from build123d import *

# Parameters (mm, degrees)
EXTRUDE_1_DEPTH      = 30
SKETCH_2_R           = 44.45
CUT_EXTRUDE_1_DEPTH  = 4
SKETCH_3_R           = 25.5
SKETCH_3_R_2         = 2.25
CUT_EXTRUDE_2_DEPTH  = 188.619295383
CUT_EXTRUDE_3_DEPTH  = 189.215302247
SKETCH_5_R           = 1.65
CUT_EXTRUDE_4_DEPTH  = 189.215302247
EXTRUDE_START        = -30
EXTRUDE_2_DEPTH      = 30
CUT_EXTRUDE_5_DEPTH  = 198.040604952
CUT_EXTRUDE_7_DEPTH  = 233.432785983
CUT_EXTRUDE_8_DEPTH  = 233.432785983
CUT_EXTRUDE_9_DEPTH  = 233.432785983
FILLET_1_R           = 5
CUT_EXTRUDE_10_DEPTH = 233.432785983
EXTRUDE_START_2      = -5
EXTRUDE_3_DEPTH      = 5
EXTRUDE_4_DEPTH      = 5
SKETCH_14_R          = 4.25
CUT_EXTRUDE_11_DEPTH = 189.364728478
SKETCH_16_W          = 43
SKETCH_16_H          = 30
CUT_EXTRUDE_12_DEPTH = 233.432785983
EXTRUDE_7_REACH      = 188.592
SKETCH_18_W          = 210
SKETCH_18_H          = 5
EXTRUDE_8_DEPTH      = 210
EXTRUDE_9_DEPTH      = 5
EXTRUDE_10_DEPTH     = 5
SKETCH_22_R          = 4.25
CUT_EXTRUDE_13_DEPTH = 187.984035343
FILLET_2_R           = 5
EXTRUDE_11_DEPTH     = 2.5
EXTRUDE_12_DEPTH     = 2.5
CUT_EXTRUDE_15_DEPTH = 5
CUT_EXTRUDE_START    = -5
CUT_EXTRUDE_16_DEPTH = 5


with BuildPart() as part:
    # 草图1 → 凸台-拉伸1 (new body)
    with BuildSketch(Plane(origin=(0, 0, 0), x_dir=(1, 0, 0), z_dir=(0, 1, 0))):
        with BuildLine():
            Line((170, 31.93), (170, -31.93))
            ThreePointArc((170, -31.93), (167.781993847, -38.210172909), (162.111885646, -41.704453387))
            Line((162.111885646, -41.704453387), (15.839142344, -73.308400404))
            ThreePointArc((15.839142344, -73.308400404), (-75, 0), (15.839142344, 73.308400404))
            Line((15.839142344, 73.308400404), (162.111885646, 41.704453387))
            ThreePointArc((162.111885646, 41.704453387), (167.781993847, 38.210172909), (170, 31.93))
        make_face()
    extrude(amount=EXTRUDE_1_DEPTH)

    # 草图2 → 切除-拉伸1 (cut)
    with BuildSketch(Plane(origin=(0, 30, 0), x_dir=(1, 0, 0), z_dir=(0, 1, 0))):
        with Locations(Location((0, 0, 0), (0, 0, 270))):
            Circle(SKETCH_2_R)
    extrude(amount=-CUT_EXTRUDE_1_DEPTH, mode=Mode.SUBTRACT)

    # 草图3 → 切除-拉伸2 (cut, through all)
    with BuildSketch(Plane(origin=(0, 26, 0), x_dir=(1, 0, 0), z_dir=(0, 1, 0))):
        with Locations(Location((0, 0, 0), (0, 0, 270))):
            Circle(SKETCH_3_R)
        with Locations(Location((0, 41, 0), (0, 0, 270))):
            Circle(SKETCH_3_R_2)
        with Locations(Location((28.991378029, 28.991378029, 0), (0, 0, 270))):
            Circle(SKETCH_3_R_2)
        with Locations(Location((41, 0, 0), (0, 0, 270))):
            Circle(SKETCH_3_R_2)
        with Locations(Location((28.991378029, -28.991378029, 0), (0, 0, 270))):
            Circle(SKETCH_3_R_2)
        with Locations(Location((0, -41, 0), (0, 0, 270))):
            Circle(SKETCH_3_R_2)
        with Locations(Location((-28.991378029, -28.991378029, 0), (0, 0, 270))):
            Circle(SKETCH_3_R_2)
        with Locations(Location((-41, 0, 0), (0, 0, 270))):
            Circle(SKETCH_3_R_2)
        with Locations(Location((-28.991378029, 28.991378029, 0), (0, 0, 270))):
            Circle(SKETCH_3_R_2)
    extrude(amount=-CUT_EXTRUDE_2_DEPTH, mode=Mode.SUBTRACT)

    # 草图4 → 切除-拉伸3 (cut, through all)
    with BuildSketch(Plane(origin=(0, 30, 0), x_dir=(1, 0, 0), z_dir=(0, 1, 0))):
        with BuildLine():
            Line((124, 18.5), (134, 18.5))
            ThreePointArc((134, 18.5), (152.5, 0), (134, -18.5))
            Line((134, -18.5), (124, -18.5))
            ThreePointArc((124, -18.5), (105.5, 0), (124, 18.5))
        make_face()
    extrude(amount=-CUT_EXTRUDE_3_DEPTH, mode=Mode.SUBTRACT)

    # 草图5 → 切除-拉伸4 (cut, through all)
    with BuildSketch(Plane(origin=(0, 30, 0), x_dir=(1, 0, 0), z_dir=(0, 1, 0))):
        with Locations(Location((116.75, 25.5, 0), (0, 0, 270))):
            Circle(SKETCH_5_R)
        with Locations(Location((141.25, 25.5, 0), (0, 0, 270))):
            Circle(SKETCH_5_R)
        with Locations(Location((141.25, -25.5, 0), (0, 0, 270))):
            Circle(SKETCH_5_R)
        with Locations(Location((116.75, -25.5, 0), (0, 0, 270))):
            Circle(SKETCH_5_R)
    extrude(amount=-CUT_EXTRUDE_4_DEPTH, mode=Mode.SUBTRACT)

    # 草图6 → 凸台-拉伸2 (add)
    with BuildSketch(Plane(origin=(0, 30, 0), x_dir=(1, 0, 0), z_dir=(0, 1, 0)).offset(EXTRUDE_START)):
        with BuildLine():
            Line((158, 95), (-52, 95))
            Line((-52, 95), (-52, 54.046276467))
            ThreePointArc((-52, 54.046276467), (-20.48558667, 72.148047366), (15.839142344, 73.308400404))
            Line((15.839142344, 73.308400404), (158, 42.592874655))
            Line((158, 42.592874655), (158, 95))
        make_face()
        with BuildLine():
            ThreePointArc((15.839142344, -73.308400404), (-20.48558667, -72.148047366), (-52, -54.046276467))
            Line((-52, -54.046276467), (-52, -95))
            Line((-52, -95), (158, -95))
            Line((158, -95), (158, -42.592874655))
            Line((158, -42.592874655), (15.839142344, -73.308400404))
        make_face()
    extrude(amount=EXTRUDE_2_DEPTH)

    # 草图7 → 切除-拉伸5 (cut, through all)
    with BuildSketch(Plane(origin=(0, 30, 0), x_dir=(1, 0, 0), z_dir=(0, 1, 0))):
        with BuildLine():
            Line((-52, 54.046276467), (-52, -54.046276467))
            ThreePointArc((-52, -54.046276467), (-75, 0), (-52, 54.046276467))
        make_face()
        with BuildLine():
            Line((158, 42.592874655), (158, -42.592874655))
            Line((158, -42.592874655), (162.111885646, -41.704453387))
            ThreePointArc((162.111885646, -41.704453387), (167.781993847, -38.210172909), (170, -31.93))
            Line((170, -31.93), (170, 31.93))
            ThreePointArc((170, 31.93), (167.781993847, 38.210172909), (162.111885646, 41.704453387))
            Line((162.111885646, 41.704453387), (158, 42.592874655))
        make_face()
    extrude(amount=-CUT_EXTRUDE_5_DEPTH, mode=Mode.SUBTRACT)

    # 草图9 → 切除-拉伸7 (cut, through all)
    with BuildSketch(Plane.ZY.offset(52)):
        Polygon((-95, 20), (-60, 10.621778265), (-60, 30), (-95, 30), align=None)
    extrude(amount=-CUT_EXTRUDE_7_DEPTH, mode=Mode.SUBTRACT)

    # 草图10 → 切除-拉伸8 (cut, through all)
    with BuildSketch(Plane.ZY.offset(52)):
        Polygon((-95, 12.753066737), (-52, 1.231251463), (-52, 0), (-95, 0), align=None)
    extrude(amount=-CUT_EXTRUDE_8_DEPTH, mode=Mode.SUBTRACT)

    # 草图8 → 切除-拉伸9 (cut, through all)
    with BuildSketch(Plane.ZY.offset(52)):
        Polygon((0, 0), (52, 0), (52, 17.3), (-52, 17.3), (-52, 0), align=None)
    extrude(amount=-CUT_EXTRUDE_9_DEPTH, mode=Mode.SUBTRACT)

    # 圆角1
    fillet_1_edges = [part.edges().sort_by_distance(p)[0] for p in [
        (53, 10.621778265, -60),
    ]]
    fillet(fillet_1_edges, radius=FILLET_1_R)

    # 草图11 → 切除-拉伸10 (cut, through all)
    with BuildSketch(Plane.ZY.offset(52)):
        Polygon((-95, 12.753066737), (-93.188266684, 19.514547521), (-95, 20), align=None)
    extrude(amount=-CUT_EXTRUDE_10_DEPTH, mode=Mode.SUBTRACT)

    # 草图12 → 凸台-拉伸3 (add)
    with BuildSketch(Plane.ZY.offset(52).offset(EXTRUDE_START_2)):
        with BuildLine():
            Line((-93.188266684, 19.514547521), (-60, 30))
            Line((-60, 30), (-60, 17.137905129))
            ThreePointArc((-60, 17.137905129), (-61.956192855, 13.171138428), (-66.294095226, 12.308275998))
            Line((-66.294095226, 12.308275998), (-93.188266684, 19.514547521))
        make_face()
    extrude(amount=EXTRUDE_3_DEPTH)

    # 草图13 → 凸台-拉伸4 (add)
    with BuildSketch(Plane(origin=(158, 0, 0), x_dir=(0, 0, -1), z_dir=(1, 0, 0))):
        with BuildLine():
            Line((66.294095226, 12.308275998), (93.188266684, 19.514547521))
            Line((93.188266684, 19.514547521), (60, 30))
            Line((60, 30), (60, 17.137905129))
            ThreePointArc((60, 17.137905129), (61.956192855, 13.171138428), (66.294095226, 12.308275998))
        make_face()
    extrude(amount=-EXTRUDE_4_DEPTH)

    # 草图14 → 切除-拉伸11 (cut, through all)
    with BuildSketch(Plane(origin=(0, -5.089745962, -1.36379332), x_dir=(1, 0, 0), z_dir=(0, 0.9659258262890681, 0.2588190451025214))):
        with Locations(Location((-27, 82.063690052, 0), (0, 0, 270))):
            Circle(SKETCH_14_R)
        with Locations(Location((23, 82.063690052, 0), (0, 0, 270))):
            Circle(SKETCH_14_R)
        with Locations(Location((83, 82.063690052, 0), (0, 0, 270))):
            Circle(SKETCH_14_R)
        with Locations(Location((133, 82.063690052, 0), (0, 0, 270))):
            Circle(SKETCH_14_R)
    extrude(amount=-CUT_EXTRUDE_11_DEPTH, mode=Mode.SUBTRACT)

    # 草图16 → 切除-拉伸12 (cut, through all)
    with BuildSketch(Plane.ZY.offset(52)):
        with Locations((73.5, 15)):
            Rectangle(SKETCH_16_W, SKETCH_16_H)
    extrude(amount=-CUT_EXTRUDE_12_DEPTH, mode=Mode.SUBTRACT)

    # 凸台-拉伸7: up to this plane
    extrude_7_end = Plane(origin=(0, -11.851226746, -3.175526636), z_dir=(0, -0.9659258262890681, -0.25881904510252146))
    # 草图18 → 凸台-拉伸7 (add, up to the surface)
    with BuildSketch(Plane(origin=(0, 30, 0), x_dir=(1, 0, 0), z_dir=(0, 1, 0)), mode=Mode.PRIVATE) as extrude_7_sk1:
        with Locations((53, -54.5)):
            Rectangle(SKETCH_18_W, SKETCH_18_H)
    extrude_7_tool1 = split(extrude(extrude_7_sk1.sketch, amount=-EXTRUDE_7_REACH, mode=Mode.PRIVATE), bisect_by=extrude_7_end, keep=Keep.BOTH, mode=Mode.PRIVATE)
    add(extrude_7_tool1.solids().sort_by_distance((53, 30, 54.5))[0])

    # 草图19 → 凸台-拉伸8 (add)
    with BuildSketch(Plane.ZY.offset(52)):
        Polygon((57, -27.975210512), (90.188266684, -36.867979769), (92, -30.106498985), (57, -20.72827725), align=None)
    extrude(amount=-EXTRUDE_8_DEPTH)

    # 草图20 → 凸台-拉伸9 (add)
    with BuildSketch(Plane.ZY.offset(52)):
        Polygon((92, -30.106498985), (57, -20.72827725), (57, 30), align=None)
    extrude(amount=-EXTRUDE_9_DEPTH)

    # 草图21 → 凸台-拉伸10 (add)
    with BuildSketch(Plane(origin=(158, 0, 0), x_dir=(0, 0, -1), z_dir=(1, 0, 0))):
        Polygon((-57, 30), (-92, -30.106498985), (-57, -20.72827725), align=None)
    extrude(amount=-EXTRUDE_10_DEPTH)

    # 草图22 → 切除-拉伸13 (cut, through all)
    with BuildSketch(Plane(origin=(0, -5.089745962, -1.36379332), x_dir=(1, 0, 0), z_dir=(0, 0.9659258262890686, 0.25881904510251946))):
        with Locations(Location((-27, -77.936309948, 0), (0, 0, 270))):
            Circle(SKETCH_22_R)
        with Locations(Location((23, -69.936309948, 0), (0, 0, 270))):
            Circle(SKETCH_22_R)
        with Locations(Location((83, -69.936309948, 0), (0, 0, 270))):
            Circle(SKETCH_22_R)
        with Locations(Location((133, -77.936309948, 0), (0, 0, 270))):
            Circle(SKETCH_22_R)
    extrude(amount=-CUT_EXTRUDE_13_DEPTH, mode=Mode.SUBTRACT)

    # 圆角2
    fillet_2_edges = [part.edges().sort_by_distance(p)[0] for p in [
        (53, -20.72827725, 57),
    ]]
    fillet(fillet_2_edges, radius=FILLET_2_R)

    # 草图25 → 凸台-拉伸11 (add, symmetric)
    with BuildSketch(Plane.ZY.offset(7.5)):
        with BuildLine():
            Line((60.705904774, -21.721271441), (92, -30.106498985))
            Line((92, -30.106498985), (57, 30))
            Line((57, 30), (57, -16.89164231))
            ThreePointArc((57, -16.89164231), (58.033233299, -19.935449455), (60.705904774, -21.721271441))
        make_face()
    extrude(amount=EXTRUDE_11_DEPTH, both=True)

    # 草图26 → 凸台-拉伸12 (add, symmetric)
    with BuildSketch(Plane(origin=(113.5, 0, 0), x_dir=(0, 0, -1), z_dir=(1, 0, 0))):
        with BuildLine():
            Line((-57, -16.89164231), (-57, 30))
            Line((-57, 30), (-92, -30.106498985))
            Line((-92, -30.106498985), (-60.705904774, -21.721271441))
            ThreePointArc((-60.705904774, -21.721271441), (-58.033233299, -19.935449455), (-57, -16.89164231))
        make_face()
    extrude(amount=EXTRUDE_12_DEPTH, both=True)

    # 草图27 → 切除-拉伸15 (cut)
    with BuildSketch(Plane(origin=(-47, 0, 0), x_dir=(0, 0, -1), z_dir=(1, 0, 0))):
        with BuildLine():
            Line((-92, -30.106498985), (-60.705904774, -21.721271441))
            ThreePointArc((-60.705904774, -21.721271441), (-58.033233299, -19.935449455), (-57, -16.89164231))
            Line((-57, -16.89164231), (-57, 30))
            Line((-57, 30), (-92, -30.106498985))
        make_face()
    extrude(amount=-CUT_EXTRUDE_15_DEPTH, mode=Mode.SUBTRACT)

    # 草图28 → 切除-拉伸16 (cut)
    with BuildSketch(Plane.ZY.offset(-153).offset(CUT_EXTRUDE_START)):
        with BuildLine():
            Line((57, 30), (57, -16.89164231))
            ThreePointArc((57, -16.89164231), (58.033233299, -19.935449455), (60.705904774, -21.721271441))
            Line((60.705904774, -21.721271441), (92, -30.106498985))
            Line((92, -30.106498985), (57, 30))
        make_face()
    extrude(amount=CUT_EXTRUDE_16_DEPTH, mode=Mode.SUBTRACT)


solid = part.part
Read the model definition and answer for the solid it produces. Units are mm, in the model's axes. A direction names the side the tool comes from. Give positions to 0.01 mm unless a question says otherwise; leave off trailing zeros. Loops run counter-clockwise (first coordinate to the right, second up) from the corner with the lowest first, then second, coordinate; pieces in that order, holes last. Notation, with made-up numbers: (38, 47) -> (91, 47) arc R15 ccw to (91, 65) -> close; hole circle Ø11 at (18, 58.5). An arc over 180 degrees is marked (long way). Use a Markdown table: item, result.
Q1. Find the intervals of material crossed by line 1 along X through (y, z) = (20, 0); line 2 along X through (y, z) = (21.5, -62.5); line 3 along X through (y, z) = (20, 41), in increasing order.
Solved:
| item | result |
|---|---|
| line 1 | x = -52 to -43.25, -38.75 to -25.5, 25.5 to 38.75, 43.25 to 105.5, 152.5 to 158 |
| line 2 | x = -52 to -47, 153 to 158 |
| line 3 | x = -52 to -2.25, 2.25 to 158 |
Q2. Section D-D, the plane z = -47.5 is taken. Determine the outline of the cut face in (x, y), then the cut area to 3 significant figures.
Solved:
| item | result |
|---|---|
| outline | (-52, 17.3) -> (158, 17.3) -> (158, 30) -> (-52, 30) -> close |
| area | 2,670 mm^2 |
Q3. Section C-C, the plane x = -34 is taken. Determine the outline of the cut face in (y, z).
Solved:
| item | result |
|---|---|
| outline | (-36.87, 90.19) -> (-26.64, 52) -> (17.3, 52) -> (17.3, -52) -> (1.23, -52) -> (12.75, -95) -> (19.51, -93.19) -> (12.31, -66.29) arc R5 cw to (17.14, -60) -> (30, -60) -> (30, -28.63) -> (26, -28.63) -> (26, 28.63) -> (30, 28.63) -> (30, 57) -> (-16.89, 57) arc R5 cw to (-21.72, 60.71) -> (-30.11, 92) -> close |
Q4. Each of these flat-tipped pins is pushed along its axis until it touches: pin 1 (12 mm diameter, centred on x = -25, y = -7.5, fed in from +Z); pin 2 (17.5 mm diameter, centred on y = -2, z = 77, fed in from +X); pin 3 (6 mm diameter, centred on x = 28.99, z = 28.99, fed in from +Y); pin 4 (2 mm diameter, centred on x = 116.75, z = 25.5, fed in from +Y). Where does it stop, or does it pass through?
Solved:
| item | result |
|---|---|
| pin 1 | stops at z = 57 |
| pin 2 | stops at x = 116 |
| pin 3 | stops at y = 26 |
| pin 4 | passes through |
Q5. Section A-A, the plane z = -12 is taken. Determine the outline of the cut face in (x, y).
Solved:
| item | result |
|---|---|
| outline | (-52, 17.3) -> (-22.5, 17.3) -> (-22.5, 26) -> (-42.8, 26) -> (-42.8, 30) -> (-52, 30) -> close; (22.5, 17.3) -> (109.92, 17.3) -> (109.92, 30) -> (42.8, 30) -> (42.8, 26) -> (22.5, 26) -> close; (148.08, 17.3) -> (158, 17.3) -> (158, 30) -> (148.08, 30) -> close |
Q6. Determine the mould class of faces 4 (the face through (53.812, -19.899, 58.006)), 5 (the face through (0.099, 21.711, 38.752)), 6 (the face through (155.535, 24.684, -76.826)) for opening direction Z: pulls with the +Z half, pulls with the -Z half, needs draft (parallel to the pull), parting line crosses it, or undercut.
Solved:
| item | result |
|---|---|
| face 4 | pulls with the +Z half |
| face 5 | undercut |
| face 6 | pulls with the -Z half |
Q7. A tool of negligible diameter and unlimited length cuts with its end or side. For faces 1 (the face through (51.6, 15.96, -79.93)), 2 (the face through (52, -4, 52)), 3 (the face through (116, -6, 67)), from which of +Z, -Z, +X, -X, +Y, -Y can it reach the whole face along a straight path? Write none if from no direction.
Solved:
| item | result |
|---|---|
| face 1 | +Y |
| face 2 | +X, -X, -Y |
| face 3 | +Z, +X, +Y |
Q8. Section B-B, the plane y = -6.5 is taken. Determine the outline of the cut face in (x, z).
Solved:
| item | result |
|---|---|
| outline | (-52, 52) -> (158, 52) -> (158, 57) -> (116, 57) -> (116, 78.25) -> (111, 78.25) -> (111, 57) -> (-5, 57) -> (-5, 78.25) -> (-10, 78.25) -> (-10, 57) -> (-52, 57) -> close |
